from build123d import *

# Parameters (mm, degrees)
F1_DEPTH = 40
F2_R     = 0.2
F3_R     = 0.5
F4_DEPTH = 50
F5_R     = 1
F6_DEPTH = 5
F7_R     = 1
F8_DEPTH = 5


with BuildPart() as f1:
    # F0 (on Top) → F1 (new body)
    with BuildSketch(Plane.XY):
        with BuildLine():
            ThreePointArc((12.489996, -0.5), (-12.5, 0), (12.489996, 0.5))
            Line((12.489996, 0.5), (13.490738, 0.5))
            ThreePointArc((13.490738, 0.5), (-13.5, 0), (13.490738, -0.5))
            Line((13.490738, -0.5), (12.489996, -0.5))
        make_face()
    extrude(amount=F1_DEPTH)

    # F2
    f2_edges = [f1.edges().sort_by_distance(p)[0] for p in [
        (13.490738, 0.5, 20),
        (12.489996, 0.5, 20),
        (12.489996, -0.5, 20),
        (13.490738, -0.5, 20),
    ]]
    fillet(f2_edges, radius=F2_R)

    # F3 (on face) → F4 (join)
    with BuildSketch(Plane.XY.offset(40)):
        with Locations((12.557036, 3.364648)):
            Circle(F3_R)
        with Locations((12.557036, -3.364648)):
            Circle(F3_R)
    extrude(amount=F4_DEPTH)

    # F5 (on face) → F6 (join)
    with BuildSketch(Plane.XY.offset(90)):
        with Locations((12.557036, -3.364648)):
            Circle(F5_R)
    extrude(amount=-F6_DEPTH)

    # F7 (on face) → F8 (join)
    with BuildSketch(Plane.XY.offset(90)):
        with Locations((12.557036, 3.364648)):
            Circle(F7_R)
    extrude(amount=-F8_DEPTH)


solid = f1.part
Can you work these out from the model? Positions are in its coordinate system, mm. A direction names the side the tool comes from. Round coordinates to 2 decimals unless told otherwise and drop trailing zeros. Order: outer loops, then holes, each group sorted by start corner. A loop starts at its lowest first (then second) coordinate and runs counter-clockwise, first axis right, second up. Notation, with made-up numbers: (72, 89) - (97, 89) arc R33 ccw to (97, 118) - close; hole circle Ø7 at (1.25, 67.25). An arc over 180 degrees is marked (long way). Answer in a Markdown table with one row per item.
(1) For P1, Ø8, axis at y = -4.5, z = 40, coming from the +X side; P2, Ø4, axis at y = -2, z = 74.5, coming from the +X side; P3, Ø2, axis at x = 6, z = 31, coming from the +Y side, each with a flat end and sliding along its axis, tell me the tip position at first contact or that it passes through.
From the geometry:
| item | result |
|---|---|
| P1 | stops at x = 13.48 |
| P2 | stops at x = 13.06 |
| P3 | stops at y = 12.54 |
(2) If we mould it in two halves opening along Y, with no side actions, what happens to faces 1 (the face through (9, -9, 0)), 2 (the face through (13.51, -3.06, 87.54)), 3 (the face through (-13.487, 0.584, 19.72))? For each: released by +Y, released by -Y, zero draft, split by the parting line, or undercut.
From the geometry:
| item | result |
|---|---|
| face 1 | zero draft |
| face 2 | undercut |
| face 3 | split by the parting line |
(3) Suppose I cut it at D-D, the plane z = 78.5. Please give me the cut outline in (x, y).
From the geometry:
| item | result |
|---|---|
| outline | circle Ø1 at (12.56, -3.36); circle Ø1 at (12.56, 3.36) |
(4) Suppose I cut it at C-C, the plane z = 24.5. Please give me the cut outline in (x, y), plus the area to 3 significant figures.
From the geometry:
| item | result |
|---|---|
| outline | (12.48, -0.69) arc R12.5 cw (long way) to (12.48, 0.69) arc R0.2 ccw to (12.68, 0.5) - (13.28, 0.5) arc R0.2 ccw to (13.48, 0.71) arc R13.5 ccw (long way) to (13.48, -0.71) arc R0.2 ccw to (13.28, -0.5) - (12.68, -0.5) arc R0.2 ccw to start |
| area | 80.6 mm2 |
(5) Suppose I cut it at A-A, the plane x = 0. Please give me the cut outline in (y, z).
From the geometry:
| item | result |
|---|---|
| outline | (-13.5, 0) - (-12.5, 0) - (-12.5, 40) - (-13.5, 40) - close; (12.5, 0) - (13.5, 0) - (13.5, 40) - (12.5, 40) - close |
(6) Please list where these lines run through material, in increasing order: L1, parallel to Y at x = 0, z = 12.5; L2, parallel to X at y = -11.5, z = 9.5; L3, parallel to Z at x = -7.25, y = 10.5. Write a range as from..to.
From the geometry:
| item | result |
|---|---|
| L1 | y = -13.5..-12.5, 12.5..13.5 |
| L2 | x = -7.07..-4.9, 4.9..7.07 |
| L3 | z = 0..40 |
(7) Suppose I cut it at B-B, the plane y = 6.5. Please give me the cut outline in (x, z), plus the area to 3 significant figures.
From the geometry:
| item | result |
|---|---|
| outline | (-11.83, 0) - (-10.68, 0) - (-10.68, 40) - (-11.83, 40) - close; (10.68, 0) - (11.83, 0) - (11.83, 40) - (10.68, 40) - close |
| area | 92.4 mm2 |
(8) Which directions (+Z, -Z, +X, -X, +Y, -Y) give clear straight access to the entire face, cutting with the end or side of a thin tool? Please do faces 4 (the face through (13.5, 3.7, 87.5)), 5 (the face through (12, -4, 85)), 6 (the face through (13, 3, 90)).
From the geometry:
| item | result |
|---|---|
| face 4 | +Z |
| face 5 | none |
| face 6 | +Z, +X, -X, +Y, -Y |
